Verification items for this drawing (mm, ordinates from the low corner). Give positions to 0.01 mm unless a question says otherwise; leave off trailing zeros. Loops run counter-clockwise (first coordinate to the right, second up) from the corner with the lowest first, then second, coordinate; pieces in that order, holes last. Notation, with made-up numbers: (39.5, 49) -> (93.5, 49) arc R24 cw to (93.5, 61) -> close; hole circle Ø5 at (61, 68.25). An arc over 180 degrees is marked (long way). Answer in a Markdown table with one row per item. Add a question column.
Q1. Material ranges on probe 1 along X at (y, z) = (33, 93) (1 decimal); probe 2 along X at (y, z) = (6.5, 55) (1 decimal); probe 3 along Z at (x, y) = (70.5, 49.5), recorded low to high.
Q2. Section check C-C on x = 100. Enter the section's corners in (y, z), and give its area (3 significant figures).
Q3. Section check A-A on y = 50. Enter the section's corners in (x, z) (1 decimal), and give its area (3 significant figures).
Q4. Section check B-B on z = 51.5. Enter the section's corners in (x, y).
Q5. Gauge pin test, flat ends, axial feed: P1, Ø8, axis at y = 31.5, z = 65.5, coming from the -X side (1 decimal); P2, Ø3, axis at x = 68, y = 11.5, coming from the +Z side (1 decimal). Record the tip position at first contact, or that the pin passes through.
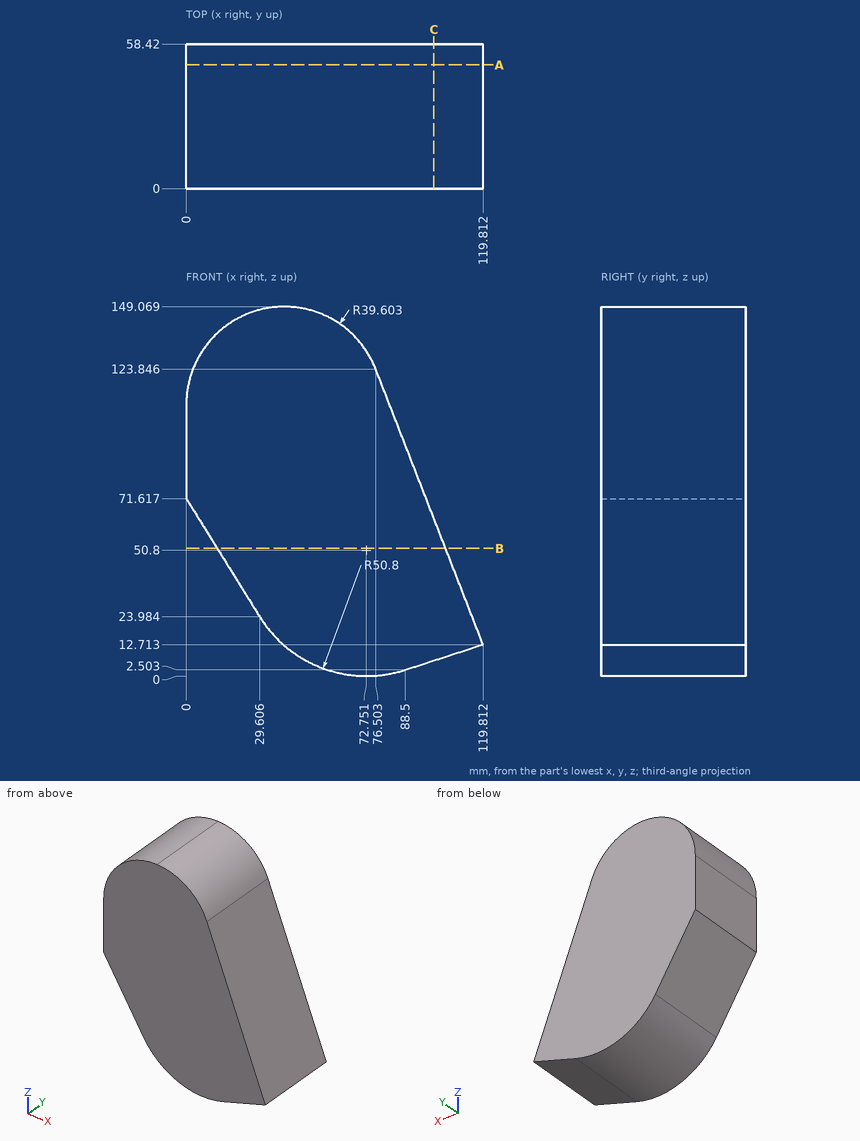
Taken from the geometry:
| question | item | result |
|---|---|---|
| 1 | probe 1 | x = 0 to 88.5 |
| 1 | probe 2 | x = 10.3 to 103.3 |
| 1 | probe 3 | z = 0.05 to 134.24 |
| 2 | outline | (0, 6.25) -> (58.42, 6.25) -> (58.42, 63.55) -> (0, 63.55) -> close |
| 2 | area | 3,350 mm² |
| 3 | outline | (0, 71.6) -> (29.6, 24) arc R50.8 ccw to (88.5, 2.5) -> (119.8, 12.7) -> (76.5, 123.8) arc R39.6 ccw to (0, 109.5) -> close |
| 3 | area | 11,800 mm² |
| 4 | outline | (12.5, 0) -> (104.7, 0) -> (104.7, 58.42) -> (12.5, 58.42) -> close |
| 5 | P1 | stops at x = 1.3 |
| 5 | P2 | stops at z = 138.5 |
